Could you check a few things on this model? Use its own coordinates, in mm. A direction names the side the tool comes from. Round coordinates to 2 decimals unless told otherwise and drop trailing zeros. Loops run counter-clockwise (first coordinate to the right, second up) from the corner with the lowest first, then second, coordinate; pieces in that order, holes last.
from build123d import *

# Parameters (mm, degrees)
SKETCH1_R                = 140
SKETCH1_R_2              = 97
BOSS_EXTRUDE1_DEPTH      = 112.5
SKETCH2_R                = 25
BOSS_EXTRUDE2_DEPTH      = 32
CIRPATTERN1_COUNT        = 3
MIRROR1_COPY_1_SKETCH_R  = 25
MIRROR1_COPY_1_DEPTH     = 32
MIRROR1_COPY_2_SKETCH_R  = 25
MIRROR1_COPY_2_DEPTH     = 32
BOSS_EXTRUDE3_REACH      = 387
BOSS_EXTRUDE3_END_RADIUS = 140
SKETCH3_R                = 100
CUT_EXTRUDE1_REACH       = 387
CUT_EXTRUDE1_END_RADIUS  = 97
SKETCH4_R                = 28
SKETCH5_R                = 50
CUT_EXTRUDE2_DEPTH       = 25
CIRPATTERN2_COUNT        = 3


with BuildPart() as part:
    # Sketch1 → Boss-Extrude1 (new body, symmetric)
    with BuildSketch(Plane(origin=(0, 0, 0), x_dir=(1, 0, 0), z_dir=(0, 1, 0))):
        with Locations(Location((0, 0, 0), (0, 0, 270))):  # turned: the seam where the file's is
            Circle(SKETCH1_R)
        with Locations(Location((0, 0, 0), (0, 0, 270))):  # turned: the seam where the file's is
            Circle(SKETCH1_R_2, mode=Mode.SUBTRACT)
    extrude(amount=BOSS_EXTRUDE1_DEPTH, both=True)

    # Sketch2 → Boss-Extrude2 (add)
    with BuildSketch(Plane(origin=(0, 112.5, 0), x_dir=(1, 0, 0), z_dir=(0, 1, 0))):
        with BuildLine():
            Line((-50, 175), (-50, 130.766968306))
            ThreePointArc((-50, 130.766968306), (0, 140), (50, 130.766968306))
            Line((50, 130.766968306), (50, 175))
            ThreePointArc((50, 175), (0, 225), (-50, 175))
        make_face()
        with Locations(Location((0, 175, 0), (0, 0, 270))):  # turned: the seam where the file's is
            Circle(SKETCH2_R, mode=Mode.SUBTRACT)
    boss_extrude2 = extrude(amount=-BOSS_EXTRUDE2_DEPTH)

    # CirPattern1: Boss-Extrude2 ×3 about axis
    cirpattern1_axis = Axis((0, 0, 0), (0, 1, 0))
    for i in range(1, CIRPATTERN1_COUNT):
        add(boss_extrude2.rotate(cirpattern1_axis, i * 360 / CIRPATTERN1_COUNT))

    # Mirror1: Boss-Extrude2 across plane
    add(boss_extrude2.mirror(Plane.ZX))

    # Mirror1 copy 1 sketch → Mirror1 copy 1 (add)
    with BuildSketch(Plane(origin=(0, -112.5, 0), x_dir=(-0.5, 0, -0.866025404), z_dir=(0, -1, 0))):
        with BuildLine():
            Line((-50, -175), (-50, -130.766968306))
            ThreePointArc((-50, -130.766968306), (0, -140), (50, -130.766968306))
            Line((50, -130.766968306), (50, -175))
            ThreePointArc((50, -175), (0, -225), (-50, -175))
        make_face()
        with Locations((0, -175)):
            Circle(MIRROR1_COPY_1_SKETCH_R, mode=Mode.SUBTRACT)
    extrude(amount=-MIRROR1_COPY_1_DEPTH)

    # Mirror1 copy 2 sketch → Mirror1 copy 2 (add)
    with BuildSketch(Plane(origin=(0, -112.5, 0), x_dir=(-0.5, 0, 0.866025404), z_dir=(0, -1, 0))):
        with BuildLine():
            Line((-50, -175), (-50, -130.766968306))
            ThreePointArc((-50, -130.766968306), (0, -140), (50, -130.766968306))
            Line((50, -130.766968306), (50, -175))
            ThreePointArc((50, -175), (0, -225), (-50, -175))
        make_face()
        with Locations((0, -175)):
            Circle(MIRROR1_COPY_2_SKETCH_R, mode=Mode.SUBTRACT)
    extrude(amount=-MIRROR1_COPY_2_DEPTH)

    # Boss-Extrude3: up to this cylinder (the profile starts outside it)
    boss_extrude3_end = Plane(origin=(0, 0, 0), z_dir=(0, -1, 0)) * Cylinder(BOSS_EXTRUDE3_END_RADIUS, 1055, mode=Mode.PRIVATE)
    # Sketch3 → Boss-Extrude3 (add, up to the surface)
    with BuildSketch(Plane.XY.offset(160), mode=Mode.PRIVATE) as boss_extrude3_sk1:
        Circle(SKETCH3_R)
    boss_extrude3_tool1 = extrude(boss_extrude3_sk1.sketch, amount=-BOSS_EXTRUDE3_REACH, mode=Mode.PRIVATE) - boss_extrude3_end
    add(boss_extrude3_tool1.solids().sort_by_distance((0, 0, 160))[0])

    # Cut-Extrude1: up to this cylinder (the profile starts outside it)
    cut_extrude1_end = Plane(origin=(0, 0, 0), z_dir=(0, -1, 0)) * Cylinder(CUT_EXTRUDE1_END_RADIUS, 969, mode=Mode.PRIVATE)
    # Sketch4 → Cut-Extrude1 (cut, up to the surface)
    with BuildSketch(Plane.XY.offset(160), mode=Mode.PRIVATE) as cut_extrude1_sk1:
        Circle(SKETCH4_R)
    cut_extrude1_tool1 = extrude(cut_extrude1_sk1.sketch, amount=-CUT_EXTRUDE1_REACH, mode=Mode.PRIVATE) - cut_extrude1_end
    add(cut_extrude1_tool1.solids().sort_by_distance((0, 0, 160))[0], mode=Mode.SUBTRACT)

    # Sketch5 → Cut-Extrude2 (cut)
    with BuildSketch(Plane.XY.offset(160)):
        Circle(SKETCH5_R)
    extrude(amount=-CUT_EXTRUDE2_DEPTH, mode=Mode.SUBTRACT)

    # Sketch7 → Ø25.0mm Dowel Hole1 (revolve, cut)
    with BuildSketch(Plane(origin=(0, 75, 160), x_dir=(0, -1, 0), z_dir=(1, 0, 0))):
        Polygon((0, 0), (0, 23.510757738), (12.5, 16), (12.5, 0), align=None)
    f_25_0mm_dowel_hole1 = revolve(axis=Axis((0, 75, 166.35), (0, 0, -1)), mode=Mode.SUBTRACT)

    # CirPattern2: Ø25.0mm Dowel Hole1 ×3 about axis
    cirpattern2_axis = Axis((0, 0, 0), (0, 0, 1))
    for i in range(1, CIRPATTERN2_COUNT):
        add(f_25_0mm_dowel_hole1.rotate(cirpattern2_axis, i * 360 / CIRPATTERN2_COUNT), mode=Mode.SUBTRACT)


solid = part.part
Item 1: If we section it at D-D, the plane z = -41.5: Please give me the cut outline in (x, y).
Results list:
outline: (-133.71, -112.5) - (-87.67, -112.5) - (-87.67, 112.5) - (-133.71, 112.5) - close; (87.67, -112.5) - (133.71, -112.5) - (133.71, 112.5) - (87.67, 112.5) - close
Item 2: If we section it at B-B, the plane x = 146.5: Please give me the cut outline in (y, z).
Results list:
outline: (-112.5, 26.85) - (-80.5, 26.85) - (-80.5, 63.02) - (-112.5, 63.02) - close; (-112.5, 111.98) - (-80.5, 111.98) - (-80.5, 137.24) - (-112.5, 137.24) - close; (80.5, 26.85) - (112.5, 26.85) - (112.5, 63.02) - (80.5, 63.02) - close; (80.5, 111.98) - (112.5, 111.98) - (112.5, 137.24) - (80.5, 137.24) - close
Item 3: If we section it at A-A, the plane z = 0: Please give me the cut outline in (x, y), then the cut area to 4 significant figures.
Results list:
outline: (-140, -112.5) - (-97, -112.5) - (-97, 112.5) - (-140, 112.5) - close; (97, -112.5) - (140, -112.5) - (140, 112.5) - (97, 112.5) - close
area: 19,350 mm2
Item 4: For faces 4 (the cylindrical face through (-27.973, 1.231, 114.23)), 5 (the flat face through (107.133, -96.724, 119.588)), 6 (the flat face through (107.133, 96.724, 119.588)), which set-ups out of +Z, -Z, +X, -X, +Y, -Y let a thin tool reach every point of the face, with its end or its side?
Results list:
face 4: +Z
face 5: +Z, -Y
face 6: +Z, +Y
Item 5: If I drill on line 1 along Y through (x, z) = (0, 149.25); line 2 along X through (y, z) = (12.5, 0); line 3 along X through (y, z) = (-37.5, 150.5), over which ranges is the centre line in solid material (lowest first)?
Results list:
line 1: y = -100 to -50, 50 to 62.5, 87.5 to 100
line 2: x = -140 to -97, 97 to 140
line 3: x = -92.7 to -77.45, -52.45 to -33.07, 33.07 to 52.45, 77.45 to 92.7
Item 6: If we section it at C-C, the plane y = 0: Please give me the cut outline in (x, z).
Results list:
outline: (-100, 97.98) arc R140 ccw (long way) to (100, 97.98) - (100, 160) - (50, 160) - (50, 135) - (28, 135) - (28, 92.87) arc R97 cw (long way) to (-28, 92.87) - (-28, 135) - (-50, 135) - (-50, 160) - (-100, 160) - close
Item 7: Will these pins go through, and if not, where does the flat tip stop? pin 1 (15 mm diameter, centred on x = 64.95, y = -37.5, fed in from +Z); pin 2 (22.5 mm diameter, centred on x = -64.95, y = -37.5, fed in from +Z); pin 3 (10 mm diameter, centred on y = 26, z = -32, fed in from -X).
Results list:
pin 1: stops at z = 141
pin 2: stops at z = 143.25
pin 3: stops at x = -137.37
Item 8: We'd pull the mould along X, two halves only. Please class faces 1 (the flat face through (179, 80.5, 90)), 2 (the cylindrical face through (-65.502, -25.012, 152.112)), 3 (the flat face through (-157.133, -96.724, 32.986)): released by +X, released by -X, zero draft, split by the parting line, or undercut.
Results list:
face 1: zero draft
face 2: undercut
face 3: released by -X
